The listing builds one solid part. Answer for the finished solid, in the listing's coordinates (mm). A direction names the side the tool comes from. Coordinates: 2 decimals unless noted, no trailing zeros. Order: outer loops, then holes, each group sorted by start corner. A loop starts at its lowest first (then second) coordinate and runs counter-clockwise, first axis right, second up. Notation, with made-up numbers: (23.25, -24.75) -> (68.25, -24.75) arc R16 ccw to (68.25, -20.75) -> close; hole circle Ø1 at (-37.75, 83.5). An arc over 180 degrees is marked (long way). Write item = value, one per line.
from build123d import *

# Parameters (mm, degrees)
CHAMFER2_SIZE      = 6
CUT_EXTRUDE2_DEPTH = 29
CHAMFER5_SIZE      = 6


with BuildPart() as part:
    # Sketch2 → Revolve2 (revolve)
    with BuildSketch(Plane.XY):
        Polygon((-16, -24.670336976), (-39, -24.670336976), (-39, 11.329663024), (-20, 11.329663024), (-20, -0.670336976), (-16, -4.670336976), align=None)
    revolve(axis=Axis((0, 25, 0), (0, -1, 0)))

    # Chamfer2
    chamfer2_edges = [part.edges().sort_by_distance(p)[0] for p in [
        (39, -24.670336976, 0),
    ]]
    chamfer(chamfer2_edges, length=CHAMFER2_SIZE)

    # Sketch8 → Cut-Extrude2 (cut, symmetric)
    with BuildSketch(Plane(origin=(0, 0, 0), x_dir=(1, 0, 0), z_dir=(0, 1, 0))):
        Polygon((3.06, 0), (0, 0), (0, -3.06), (-3.06, -3.06), (-3.06, -23.05), (3.06, -23.05), align=None)
        Polygon((-3.06, -3.06), (-3.06, 0), (0, 0), (0, 3.06), (-24.04, 3.06), (-24.04, -3.06), align=None)
    extrude(amount=CUT_EXTRUDE2_DEPTH, both=True, mode=Mode.SUBTRACT)

    # Chamfer5
    chamfer5_edges = [part.edges().sort_by_distance(p)[0] for p in [
        (39, 11.329663024, 0),
    ]]
    chamfer(chamfer5_edges, length=CHAMFER5_SIZE)


solid = part.part
Q1. Section B-B, the plane z = 0 is taken. Give the vertices of the cut face in (x, y).
The answers:
outline = (-39, -18.67) -> (-33, -24.67) -> (-24.04, -24.67) -> (-24.04, 11.33) -> (-33, 11.33) -> (-39, 5.33) -> close; (16, -24.67) -> (33, -24.67) -> (39, -18.67) -> (39, 5.33) -> (33, 11.33) -> (20, 11.33) -> (20, -0.67) -> (16, -4.67) -> close
Q2. Section A-A, the plane x = 0 is taken. Give the vertices of the cut face in (y, z), plus the area to 3 significant figures.
The answers:
outline = (-24.67, -33) -> (-18.67, -39) -> (5.33, -39) -> (11.33, -33) -> (11.33, -20) -> (-0.67, -20) -> (-4.67, -16) -> (-24.67, -16) -> close; (-24.67, 23.05) -> (11.33, 23.05) -> (11.33, 33) -> (5.33, 39) -> (-18.67, 39) -> (-24.67, 33) -> close
area = 1,270 mm2
Q3. Find the intervals of material crossed by line 1 along Z through (x, y) = (0, -9.75); line 2 along X through (y, z) = (-14.5, 0); line 3 along Z through (x, y) = (6.5, -7.5), in increasing order.
The answers:
line_1 = -39 to -16, 23.05 to 39
line_2 = -39 to -24.04, 16 to 39
line_3 = -38.45 to -14.62, 14.62 to 38.45
Q4. A tool of negligible diameter and unlimited length cuts with its end or side. For faces 1 (the face through (15, 11.33, 14)), 2 (the face through (3.06, -10, 20)), 3 (the face through (-12.284, -3.143, 12.503)), from which of +Z, -Z, +X, -X, +Y, -Y can it reach the whole face along a straight path? Write none if from no direction.
The answers:
face_1 = +Z, -Z, +X, -X, +Y
face_2 = +Y, -Y
face_3 = +Y
Q5. The mould has two halves that part along Z. Classify faces 4 (the face through (33.26, 11.04, -1.46)), 5 (the face through (14.2, -24.67, -7.8)), 6 (the face through (10.97, -14.81, -11.65)): released by +Z, released by -Z, zero draft, split by the parting line, or undercut.
The answers:
face_4 = split by the parting line
face_5 = zero draft
face_6 = undercut
Q6. Section C-C, the plane y = 3 is taken. Give the vertices of the cut face in (x, z), plus the area to 3 significant figures.
The answers:
outline = circle Ø78 at (0, 0); hole (-24.04, -3.06) -> (-19.76, -3.06) arc R20 ccw (long way) to (3.06, 19.76) -> (3.06, 23.05) -> (-3.06, 23.05) -> (-3.06, 19.76) arc R20 ccw to (-19.76, 3.06) -> (-24.04, 3.06) -> close
area = 3,480 mm2
Q7. Each of these flat-tipped pins is pushed along its axis until it touches: pin 1 Ø5 at (x, y) = (1, -8.5) entering from -Z; pin 2 Ø2 at (y, z) = (3.5, 23) entering from +X; pin 3 Ø3 at (x, y) = (-16.5, -18.5) entering from -Z. Where does it stop, or does it pass through?
The answers:
pin_1 = -39
pin_2 = 32.2
pin_3 = -36
